```python
from build123d import *

# Parameters (mm, degrees)
BOSS_EXTRUDE1_DEPTH = 24.61
SKETCH2_R           = 4
CUT_EXTRUDE5_DEPTH  = 20
SKETCH4_R           = 1.09
CUT_EXTRUDE6_DEPTH  = 100
CIRPATTERN1_COUNT   = 4
SKETCH5_R           = 4
CUT_EXTRUDE7_DEPTH  = 50
SKETCH6_R           = 1.09
CUT_EXTRUDE8_DEPTH  = 50
CIRPATTERN2_COUNT   = 4
FILLET1_R           = 1
SKETCH7_W           = 24.61
SKETCH7_H           = 17.78
CUT_EXTRUDE9_DEPTH  = 100


with BuildPart() as part:
    # Sketch1 → Boss-Extrude1 (new body)
    with BuildSketch(Plane.XY):
        Polygon((-26.125, 58.34), (-26.125, 0), (26.125, 0), (26.125, 58.34), (24.605, 58.34), (24.605, 1.52), (-24.605, 1.52), (-24.605, 58.34), align=None)
    extrude(amount=BOSS_EXTRUDE1_DEPTH)

    # Sketch2 → Cut-Extrude5 (cut)
    with BuildSketch(Plane.ZY.offset(26.125)):
        with Locations(Location((12.305, 28.28, 0), (0, 0, 270))):
            Circle(SKETCH2_R)
        with BuildLine():
            Line((-0.005, 28.28), (-0.002957418, 40.56))
            Line((-0.002957418, 40.56), (11.446105362, 40.56))
            ThreePointArc((11.446105362, 40.56), (3.301970149, 36.675329267), (-0.005, 28.28))
        make_face()
        with BuildLine():
            Line((24.612957418, 40.56), (24.615, 28.28))
            ThreePointArc((24.615, 28.28), (21.308029851, 36.675329267), (13.163894638, 40.56))
            Line((13.163894638, 40.56), (24.612957418, 40.56))
        make_face()
    cut_extrude5 = extrude(amount=-CUT_EXTRUDE5_DEPTH, mode=Mode.SUBTRACT)

    # Mirror1: Cut-Extrude5 across plane
    add(cut_extrude5.mirror(Plane(origin=(0, 0, 0), x_dir=(0, 0, 1), z_dir=(1, 0, 0))), mode=Mode.SUBTRACT)

    # Sketch4 → Cut-Extrude6 (cut)
    with BuildSketch(Plane.ZY.offset(26.125)):
        with Locations(Location((12.305, 36.78, 0), (0, 0, 270))):
            Circle(SKETCH4_R)
    cut_extrude6 = extrude(amount=-CUT_EXTRUDE6_DEPTH, mode=Mode.SUBTRACT)

    # CirPattern1: Cut-Extrude6 ×4 about axis
    cirpattern1_axis = Axis((0, 28.28, 12.305), (1, 0, 0))
    for i in range(1, CIRPATTERN1_COUNT):
        add(cut_extrude6.rotate(cirpattern1_axis, i * 360 / CIRPATTERN1_COUNT), mode=Mode.SUBTRACT)

    # Sketch5 → Cut-Extrude7 (cut, symmetric)
    with BuildSketch(Plane(origin=(0, 1.52, 0), x_dir=(1, 0, 0), z_dir=(0, 1, 0))):
        with Locations(Location((0, -12.305, 0), (0, 0, 270))):
            Circle(SKETCH5_R)
    extrude(amount=CUT_EXTRUDE7_DEPTH, both=True, mode=Mode.SUBTRACT)

    # Sketch6 → Cut-Extrude8 (cut, symmetric)
    with BuildSketch(Plane(origin=(0, 1.52, 0), x_dir=(1, 0, 0), z_dir=(0, 1, 0))):
        with Locations(Location((0, -3.805, 0), (0, 0, 270))):
            Circle(SKETCH6_R)
    cut_extrude8 = extrude(amount=CUT_EXTRUDE8_DEPTH, both=True, mode=Mode.SUBTRACT)

    # CirPattern2: Cut-Extrude8 ×4 about axis
    cirpattern2_axis = Axis((0, 0, 12.305), (0, 1, 0))
    for i in range(1, CIRPATTERN2_COUNT):
        add(cut_extrude8.rotate(cirpattern2_axis, i * 360 / CIRPATTERN2_COUNT), mode=Mode.SUBTRACT)

    # Fillet1
    fillet1_edges = [part.edges().sort_by_distance(p)[0] for p in [
        (-24.605, 1.52, 12.305),
        (24.605, 1.52, 12.305),
        (26.125, 0, 12.305),
        (-26.125, 0, 12.305),
    ]]
    fillet(fillet1_edges, radius=FILLET1_R)

    # Sketch7 → Cut-Extrude9 (cut)
    with BuildSketch(Plane.ZY.offset(26.125)):
        with Locations((12.305, 49.45)):
            Rectangle(SKETCH7_W, SKETCH7_H)
    extrude(amount=-CUT_EXTRUDE9_DEPTH, mode=Mode.SUBTRACT)


solid = part.part
```
Geometry check sheet. Reference: the model listing, model coordinates, mm. A direction names the side the tool comes from. Coordinates: 2 decimals unless noted, no trailing zeros. Loops run counter-clockwise (first coordinate to the right, second up) from the corner with the lowest first, then second, coordinate; pieces in that order, holes last.
Item 1: Sectioned sample at D-D, the plane x = 0. Record the boundary of the cut face in (y, z) (3 decimals).
Item 2: Sectioned sample at B-B, the plane z = 3.5. Record the boundary of the cut face in (x, y) (3 decimals), then the cut area to 3 significant figures.
Item 3: Sectioned sample at A-A, the plane x = 8.5. Record the boundary of the cut face in (y, z) (3 decimals), then the cut area to 3 significant figures.
Item 4: Thickness scan on line 1 (X direction, y = 26, z = 17.75) (3 decimals); line 2 (Z direction, x = 25, y = 28); line 3 (Y direction, x = -6, z = 15.25). Record the ranges inside material, lowest first.
Item 5: Go/stop test with flat-tipped pins: pin 1 Ø6.5 at (x, z) = (0, 12.305) entering from +Y; pin 2 Ø4 at (x, z) = (16, 7) entering from +Y. Record where each tip stops, or that it passes through.
Item 6: Sectioned sample at C-C, the plane y = 19.78. Record the boundary of the cut face in (x, z) (3 decimals).
Item 7: Release check for a two-part mould opening along Z. For faces 1 (the face through (-25.376, 32.276, 12.481)), 2 (the face through (25.376, 36.711, 21.275)), 3 (the face through (25.376, 36.894, 3.511)) record: released by +Z, released by -Z, zero draft, split by the parting line, or undercut.
Item 8: Access from +Z, -Z, +X, -X, +Y, -Y to the whole of each face (thin tool, end or side, straight path). Record for faces 4 (the face through (25.35, 20.82, 11.98)), 5 (the face through (24.605, 22, 12)).
Check result:
1. outline: (0, 0) - (1.52, 0) - (1.52, 2.715) - (0, 2.715) - close; (0, 4.895) - (1.52, 4.895) - (1.52, 8.305) - (0, 8.305) - close; (0, 16.305) - (1.52, 16.305) - (1.52, 19.715) - (0, 19.715) - close; (0, 21.895) - (1.52, 21.895) - (1.52, 24.61) - (0, 24.61) - close
2. outline: (-26.125, 1) arc R1 ccw to (-25.125, 0) - (-1.046, 0) - (-1.046, 1.52) - (-23.605, 1.52) arc R1 cw to (-24.605, 2.52) - (-24.605, 27.234) - (-26.125, 27.234) - close; (-26.125, 29.326) - (-24.605, 29.326) - (-24.605, 36.883) - (-26.125, 36.883) - close; (1.046, 0) - (25.125, 0) arc R1 ccw to (26.125, 1) - (26.125, 27.234) - (24.605, 27.234) - (24.605, 2.52) arc R1 cw to (23.605, 1.52) - (1.046, 1.52) - close; (24.605, 29.326) - (26.125, 29.326) - (26.125, 36.883) - (24.605, 36.883) - close
2. area: 177 mm2
3. outline: (0, 0) - (1.52, 0) - (1.52, 11.215) - (0, 11.215) - close; (0, 13.395) - (1.52, 13.395) - (1.52, 24.61) - (0, 24.61) - close
3. area: 34.1 mm2
4. line 1: x = -26.125 to -24.605, 24.605 to 26.125
4. line 2: z = 0 to 2.75, 4.86 to 8.31, 16.3 to 19.75, 21.86 to 24.61
4. line 3: y = 0 to 1.52
5. pin 1: passes through
5. pin 2: stops at y = 1.52
6. outline: (-26.125, 0) - (-24.605, 0) - (-24.605, 11.215) - (-26.125, 11.215) - close; (-26.125, 13.395) - (-24.605, 13.395) - (-24.605, 24.61) - (-26.125, 24.61) - close; (24.605, 0) - (26.125, 0) - (26.125, 11.215) - (24.605, 11.215) - close; (24.605, 13.395) - (26.125, 13.395) - (26.125, 24.61) - (24.605, 24.61) - close
7. face 1: undercut
7. face 2: released by +Z
7. face 3: released by -Z
8. face 4: +X, -X
8. face 5: +Z, -Z, +Y
